For this review, take the finished solid that the model builds, in its own axes (mm). Coordinates: 2 decimals unless noted, no trailing zeros. Loops run counter-clockwise (first coordinate to the right, second up) from the corner with the lowest first, then second, coordinate; pieces in that order, holes last.
1. Take a section at B-B, the plane z = -2.5. State the section outline as (x, y) points.
2. Take a section at A-A, the plane x = 0. State the section outline as (y, z) points, then the cut area to 3 significant figures.
3. To check wall thickness, follow probe 1 along X at (y, z) = (1.5, 0); probe 2 along Z at (x, y) = (0.5, 1.05); probe 3 along X at (y, z) = (1.9, 6.75). State the ranges of each line that lie inside material, in increasing order.
4. Take a section at D-D, the plane y = 1.65. Count the separate pieces of the cut face and the enclosed holes in it, then the cut area to 3 significant figures.
5. Take a section at C-C, the plane x = -10.5. State the section outline as (y, z) points, then the cut area to 3 significant figures.
6. Clearance check with flat-ended pins moving along their axes: P1, Ø5, axis at x = 11.69, z = -6.75, coming from the +Y side; P2, Ø1.5, axis at y = 0.5, z = 2, coming from the +X side; P3, Ø1, axis at y = 0.5, z = -5.5, coming from the -X side; P4, Ø1.5, axis at x = -13, y = 1.5, coming from the +Z side. State where each tip first meets the part, or that it passes through.
```python
from build123d import *

# Parameters (mm, degrees)
SKETCH_1_R          = 18
SKETCH_1_R_2        = 1.6
SKETCH_1_R_3        = 2
EXTRUDE_1_DEPTH     = 3
SKETCH_3_R          = 4.75
CUT_EXTRUDE_1_DEPTH = 4


with BuildPart() as part:
    # 草图1 → 凸台-拉伸1 (new body)
    with BuildSketch(Plane(origin=(0, 0, 0), x_dir=(1, 0, 0), z_dir=(0, 1, 0))):
        with Locations(Location((0, 0, 0), (0, 0, 270))):
            Circle(SKETCH_1_R)
        with Locations(Location((0, 13.5, 0), (0, 0, 270))):
            Circle(SKETCH_1_R_2, mode=Mode.SUBTRACT)
        with Locations(Location((11.691342951, 6.75, 0), (0, 0, 270))):
            Circle(SKETCH_1_R_2, mode=Mode.SUBTRACT)
        with Locations(Location((11.691342951, -6.75, 0), (0, 0, 270))):
            Circle(SKETCH_1_R_2, mode=Mode.SUBTRACT)
        with Locations(Location((0, -13.5, 0), (0, 0, 270))):
            Circle(SKETCH_1_R_2, mode=Mode.SUBTRACT)
        with Locations(Location((-11.691342951, -6.75, 0), (0, 0, 270))):
            Circle(SKETCH_1_R_2, mode=Mode.SUBTRACT)
        with Locations(Location((-11.691342951, 6.75, 0), (0, 0, 270))):
            Circle(SKETCH_1_R_2, mode=Mode.SUBTRACT)
        with Locations(Location((12, 0, 0), (0, 0, 270))):
            Circle(SKETCH_1_R_3, mode=Mode.SUBTRACT)
        with Locations(Location((-6, -10.392304845, 0), (0, 0, 270))):
            Circle(SKETCH_1_R_3, mode=Mode.SUBTRACT)
        with Locations(Location((-6, 10.392304845, 0), (0, 0, 270))):
            Circle(SKETCH_1_R_3, mode=Mode.SUBTRACT)
    extrude(amount=EXTRUDE_1_DEPTH)

    # 草图3 → 切除-拉伸1 (cut)
    with BuildSketch(Plane(origin=(0, 3, 0), x_dir=(1, 0, 0), z_dir=(0, 1, 0))):
        with Locations(Location((0, 0, 0), (0, 0, 270))):
            Circle(SKETCH_3_R)
    extrude(amount=-CUT_EXTRUDE_1_DEPTH, mode=Mode.SUBTRACT)


solid = part.part
```
Results list:
1. outline: (-17.83, 0) - (-4.04, 0) - (-4.04, 3) - (-17.83, 3) - close; (4.04, 0) - (17.83, 0) - (17.83, 3) - (4.04, 3) - close
2. outline: (0, -18) - (3, -18) - (3, -15.1) - (0, -15.1) - close; (0, -11.9) - (3, -11.9) - (3, -4.75) - (0, -4.75) - close; (0, 4.75) - (3, 4.75) - (3, 11.9) - (0, 11.9) - close; (0, 15.1) - (3, 15.1) - (3, 18) - (0, 18) - close
2. area: 60.3 mm2
3. probe 1: x = -18 to -4.75, 4.75 to 10, 14 to 18
3. probe 2: z = -17.99 to -15.02, -11.98 to -4.72, 4.72 to 11.98, 15.02 to 17.99
3. probe 3: x = -16.69 to -13.29, -10.09 to 10.09, 13.29 to 16.69
4. separate pieces: 1
4. enclosed holes: 10
4. area: 861 mm2
5. outline: (0, -14.62) - (3, -14.62) - (3, -7.82) - (0, -7.82) - close; (0, -5.68) - (3, -5.68) - (3, 5.68) - (0, 5.68) - close; (0, 7.82) - (3, 7.82) - (3, 14.62) - (0, 14.62) - close
5. area: 74.9 mm2
6. P1: stops at y = 3
6. P2: stops at x = 17.96
6. P3: stops at x = -17.29
6. P4: stops at z = 13.19
